```python
from build123d import *

# Parameters (mm, degrees)
F1_DEPTH       = 2
F2_R           = 2.5
F2_R_2         = 1.5
F3_DEPTH       = 2
F5_DEPTH       = 4
F7_D           = 3
F7_CBORE_D     = 5
F7_CBORE_DEPTH = 0.5


with BuildPart() as f1:
    # F0 (on Top) → F1 (new body)
    with BuildSketch(Plane.XY):
        with BuildLine():
            Line((-174.5, -132.5), (174.5, -132.5))
            ThreePointArc((174.5, -132.5), (176.62132, -131.62132), (177.5, -129.5))
            Line((177.5, -129.5), (177.5, 129.5))
            ThreePointArc((177.5, 129.5), (176.62132, 131.62132), (174.5, 132.5))
            Line((174.5, 132.5), (-174.5, 132.5))
            ThreePointArc((-174.5, 132.5), (-176.62132, 131.62132), (-177.5, 129.5))
            Line((-177.5, 129.5), (-177.5, -129.5))
            ThreePointArc((-177.5, -129.5), (-176.62132, -131.62132), (-174.5, -132.5))
        make_face()
    extrude(amount=F1_DEPTH)

    # F2 (on face) → F3 (join)
    with BuildSketch(Plane.XY.offset(2)):
        with Locations((-169.5, 127.5)):
            Circle(F2_R)
        with Locations((-169.5, 127.5)):
            Circle(F2_R_2, mode=Mode.SUBTRACT)
        with Locations((168, 127.5)):
            Circle(F2_R)
        with Locations((168, 127.5)):
            Circle(F2_R_2, mode=Mode.SUBTRACT)
        with Locations((-169.5, -117.5)):
            Circle(F2_R)
        with Locations((-169.5, -117.5)):
            Circle(F2_R_2, mode=Mode.SUBTRACT)
        with Locations((168, -117.5)):
            Circle(F2_R)
        with Locations((168, -117.5)):
            Circle(F2_R_2, mode=Mode.SUBTRACT)
    extrude(amount=F3_DEPTH)

    # F4 (on face) → F5 (join)
    with BuildSketch(Plane.XY.offset(2)):
        with BuildLine():
            Line((174.5, 132.5), (-174.5, 132.5))
            ThreePointArc((-174.5, 132.5), (-176.62132, 131.62132), (-177.5, 129.5))
            Line((-177.5, 129.5), (-177.5, -129.5))
            ThreePointArc((-177.5, -129.5), (-176.62132, -131.62132), (-174.5, -132.5))
            Line((-174.5, -132.5), (174.5, -132.5))
            ThreePointArc((174.5, -132.5), (176.62132, -131.62132), (177.5, -129.5))
            Line((177.5, -129.5), (177.5, 129.5))
            ThreePointArc((177.5, 129.5), (176.62132, 131.62132), (174.5, 132.5))
        make_face()
        with BuildLine():
            ThreePointArc((-176.5, 129.5), (-175.914214, 130.914214), (-174.5, 131.5))
            Line((-174.5, 131.5), (174.5, 131.5))
            ThreePointArc((174.5, 131.5), (175.914214, 130.914214), (176.5, 129.5))
            Line((176.5, 129.5), (176.5, -129.5))
            ThreePointArc((176.5, -129.5), (175.914214, -130.914214), (174.5, -131.5))
            Line((174.5, -131.5), (-174.5, -131.5))
            ThreePointArc((-174.5, -131.5), (-175.914214, -130.914214), (-176.5, -129.5))
            Line((-176.5, -129.5), (-176.5, 129.5))
        make_face(mode=Mode.SUBTRACT)
    extrude(amount=F5_DEPTH)

    # F7 (through all)
    with Locations(Plane(origin=(0, 0, 0), x_dir=(1, 0, 0), z_dir=(0, 0, -1))):
        with Locations((-169.5, -127.5), (168, -127.5), (168, 117.5), (-169.5, 117.5)):
            CounterBoreHole(F7_D / 2, F7_CBORE_D / 2, F7_CBORE_DEPTH)


solid = f1.part
```
Check sheet for the modelled part. Datum: model origin and axes. Units: mm. Round coordinates to 2 decimals unless told otherwise and drop trailing zeros. Order: outer loops, then holes, each group sorted by start corner. A loop starts at its lowest first (then second) coordinate and runs counter-clockwise, first axis right, second up. Notation, with made-up numbers: M 14,-16.75 L 55,-16.75 A20 ccw 55,11.25 Z; hole C 23,39 d3. An arc over 180 degrees is marked long. Answer in a Markdown table with one row per item.
(1) Material ranges on line 1 along Y through (x, z) = (168, 1.5); line 2 along X through (y, z) = (127.5, 0.35); line 3 along X through (y, z) = (-14, 2.8), recorded low to high. Write a range as from..to.
Findings:
| item | result |
|---|---|
| line 1 | y = -132.5..-119, -116..126, 129..132.5 |
| line 2 | x = -177.5..-172, -167..165.5, 170.5..177.5 |
| line 3 | x = -177.5..-176.5, 176.5..177.5 |
(2) Gauge pin test, flat ends, axial feed: pin 1 (6.5 mm diameter, centred on x = 168, y = -117.5, fed in from +Z); pin 2 (6 mm diameter, centred on x = -94.5, y = 91.5, fed in from +Z). Record the tip position at first contact, or that the pin passes through.
Findings:
| item | result |
|---|---|
| pin 1 | stops at z = 4 |
| pin 2 | stops at z = 2 |
(3) Draft check along Y on faces 1 (the flat face through (-2, 2, 2)), 2 (the flat face through (-2, 2, 0)). Enter one of: +Y half, -Y half, draft (parallel to the pull), parting line (faces both ways), or undercut.
Findings:
| item | result |
|---|---|
| face 1 | undercut |
| face 2 | draft |
(4) Section check A-A on y = -62.5. Record the boundary of the cut face in (x, z), plus the area to 3 significant figures.
Findings:
| item | result |
|---|---|
| outline | M -177.5,0 L 177.5,0 L 177.5,6 L 176.5,6 L 176.5,2 L -176.5,2 L -176.5,6 L -177.5,6 Z |
| area | 718 mm^2 |
(5) Section check B-B on x = 3.5. Record the boundary of the cut face in (y, z), plus the area to 3 significant figures.
Findings:
| item | result |
|---|---|
| outline | M -132.5,0 L 132.5,0 L 132.5,6 L 131.5,6 L 131.5,2 L -131.5,2 L -131.5,6 L -132.5,6 Z |
| area | 538 mm^2 |
